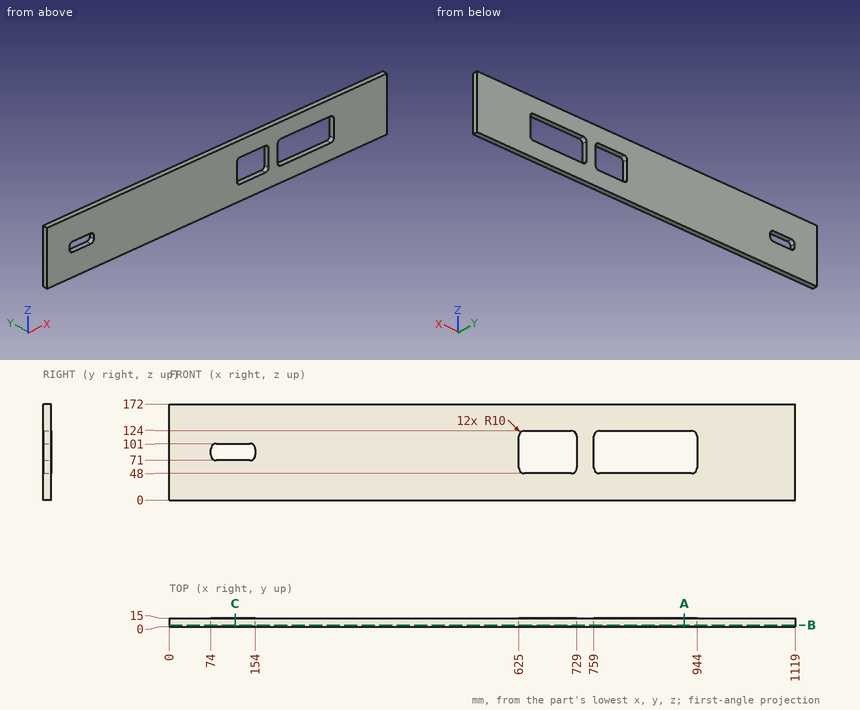
For this review, use the dimensioned drawing (mm, ordinates from the lowest corner) and the shaded views. Coordinates: 2 decimals unless noted, no trailing zeros. Loops run counter-clockwise (first coordinate to the right, second up) from the corner with the lowest first, then second, coordinate; pieces in that order, holes last. Notation, with made-up numbers: M -29,-6 L 10,-6 A15 ccw 10,3 Z; hole C 23,59.5 d2. An arc over 180 degrees is marked long. Answer as CSV lines item,"result".
Item 1: Add section A-A on x = 921. State the section outline as (y, z) points, plus the area to 3 significant figures.
Answer list:
outline,"M 0,0 L 15,0 L 15,48 L 0,48 Z; M 0,124 L 15,124 L 15,172 L 0,172 Z"
area,"1,440 mm²"
Item 2: For probe 1 along X at (y, z) = (8.25, 63.5); probe 2 along X at (y, z) = (5.5, 84); probe 3 along Z at (x, y) = (683.5, 2.5), list the stretches that pass through material, from the lowest coordinate up.
Answer list:
probe 1,"0 to 625, 729 to 759, 944 to 1119"
probe 2,"0 to 74, 154 to 625, 729 to 759, 944 to 1119"
probe 3,"0 to 48, 124 to 172"
Item 3: Add section B-B on y = 2.5. State the section outline as (x, z) points, plus the area to 3 significant figures.
Answer list:
outline,"M 0,0 L 1119,0 L 1119,172 L 0,172 Z; hole M 74,81 A10 ccw 84,71 L 144,71 A10 ccw 154,81 L 154,91 A10 ccw 144,101 L 84,101 A10 ccw 74,91 Z; hole M 625,58 A10 ccw 635,48 L 719,48 A10 ccw 729,58 L 729,114 A10 ccw 719,124 L 635,124 A10 ccw 625,114 Z; hole M 759,58 A10 ccw 769,48 L 934,48 A10 ccw 944,58 L 944,114 A10 ccw 934,124 L 769,124 A10 ccw 759,114 Z"
area,"168,000 mm²"
Item 4: Add section C-C on x = 117.5. State the section outline as (y, z) points, plus the area to 3 significant figures.
Answer list:
outline,"M 0,0 L 15,0 L 15,71 L 0,71 Z; M 0,101 L 15,101 L 15,172 L 0,172 Z"
area,"2,130 mm²"
